from build123d import *

# Parameters (mm, degrees)
F0_W     = 254
F0_H     = 254
F1_DEPTH = 38.1
F2_SIZE  = 12.7
F3_R     = 21.5591889527
F4_DEPTH = 38.1
F5_W     = 101.6
F5_H     = 50.8
F6_DEPTH = 3.175
F7_W     = 88.9000004845
F7_H     = 38.1000004845
F8_DEPTH = 38.101
F9_R     = 5.08
F10_SIZE = 12.7


with BuildPart() as f1:
    # F0 (on Top) → F1 (new body)
    with BuildSketch(Plane.XY):
        Rectangle(F0_W, F0_H)
    extrude(amount=F1_DEPTH)

    # F2
    f2_edges = [f1.edges().sort_by_distance(p)[0] for p in [
        (-127, -127, 19.05),
        (127, -127, 19.05),
        (-127, 127, 19.05),
        (127, 127, 19.05),
    ]]
    chamfer(f2_edges, length=F2_SIZE)

    # F3 (on face) → F4 (cut, through all)
    with BuildSketch(Plane.XY.offset(38.1)):
        with Locations((0, 50.8)):
            Circle(F3_R)
    extrude(amount=-F4_DEPTH, mode=Mode.SUBTRACT)

    # F5 (on face) → F6 (cut)
    with BuildSketch(Plane.XY.offset(38.1)):
        with Locations((0, -68.0069606819)):
            Rectangle(F5_W, F5_H)
    extrude(amount=-F6_DEPTH, mode=Mode.SUBTRACT)

    # F7 (on face) → F8 (cut, through all)
    with BuildSketch(Plane.XY.offset(38.1)):
        with Locations((0, -68.0069606819)):
            Rectangle(F7_W, F7_H)
    extrude(amount=-F8_DEPTH, mode=Mode.SUBTRACT)

    # F9
    f9_edges = [f1.edges().sort_by_distance(p)[0] for p in [
        (-50.8, -42.606961, 36.5125),
        (-44.45, -48.95696, 17.4625),
        (44.45, -48.95696, 17.4625),
        (50.8, -42.606961, 36.5125),
        (50.8, -93.406961, 36.5125),
        (44.45, -87.056961, 17.4625),
        (-44.45, -87.056961, 17.4625),
        (-50.8, -93.406961, 36.5125),
    ]]
    fillet(f9_edges, radius=F9_R)

    # F10
    f10_edges = [f1.edges().sort_by_distance(p)[0] for p in [
        (0, -127, 38.1),
        (-120.65, -120.65, 38.1),
        (-127, 0, 38.1),
        (-120.65, 120.65, 38.1),
        (0, 127, 38.1),
        (120.65, 120.65, 38.1),
        (120.65, -120.65, 38.1),
        (127, 0, 38.1),
    ]]
    chamfer(f10_edges, length=F10_SIZE)


solid = f1.part
Here's how the part is built. I have some questions about the finished solid (model axes, mm). A direction names the side the tool comes from. Round coordinates to 2 decimals unless told otherwise and drop trailing zeros. Write each loop counter-clockwise with the first axis right and the second up, starting at its lowest first coordinate (ties: lowest second). Pieces come first, ordered by that corner, then holes.
1. Suppose I cut it at B-B (x = 0). List the corners of the cut face in (y, z) for me (3 decimals), and give its area (3 significant figures).
2. Suppose I cut it at D-D (x = -82.5). List the corners of the cut face in (y, z) for me, and give its area (3 significant figures).
3. I need wall thicknesses on L1, parallel to Y at x = 0, z = 9; L2, parallel to X at y = 50, z = 21; L3, parallel to Y at x = 27, z = 6. Which ranges of each line are inside material? Lowest first, please.
4. For faces 4 (the flat face through (-44.45, -68, 18)), 5 (the flat face through (0, -47, 34.925)), 6 (the flat face through (120.7, -120.6, 12.5)), which set-ups out of +Z, -Z, +X, -X, +Y, -Y let a thin tool reach every point of the face, with its end or its side?
5. Will these pins go through, and if not, where does the flat tip stop? pin 1 Ø1.6 at (y, z) = (-77, 36.5) entering from -X; pin 2 Ø2.5 at (x, z) = (-5.5, 37) entering from -Y; pin 3 Ø3.5 at (x, z) = (-20, 36.5) entering from +Y.
6. If we mould it in two halves opening along X, with no side actions, what happens to faces 1 (the flat face through (-2, 2, 0)), 2 (the flat face through (-127, -2, 13)), 3 (the flat face through (44.45, -68, 18))? For each: released by +X, released by -X, zero draft, split by the parting line, or undercut.
7. Suppose I cut it at C-C (z = 22). List the corners of the cut face in (x, y) for me.
8. Suppose I cut it at A-A (y = 50.8). List the corners of the cut face in (x, z) for me.
Answer sheet:
1. outline: (-127, 0) - (-87.057, 0) - (-87.057, 34.925) - (-93.407, 34.925) - (-93.407, 38.1) - (-114.3, 38.1) - (-127, 25.4) - close; (-48.957, 0) - (29.241, 0) - (29.241, 38.1) - (-42.607, 38.1) - (-42.607, 34.925) - (-48.957, 34.925) - close; (72.359, 0) - (127, 0) - (127, 25.4) - (114.3, 38.1) - (72.359, 38.1) - close
1. area: 6,380 mm2
2. outline: (-127, 0) - (127, 0) - (127, 25.4) - (114.3, 38.1) - (-114.3, 38.1) - (-127, 25.4) - close
2. area: 9,520 mm2
3. L1: y = -127 to -87.06, -48.96 to 29.24, 72.36 to 127
3. L2: x = -127 to -21.54, 21.54 to 127
3. L3: y = -127 to -87.06, -48.96 to 127
4. face 4: +Z, -Z
4. face 5: +Z
4. face 6: +Z, -Z, +X, -Y
5. pin 1: stops at x = -116.7
5. pin 2: stops at y = -116.65
5. pin 3: stops at y = 117.65
6. face 1: zero draft
6. face 2: released by -X
6. face 3: undercut
7. outline: (-127, -114.3) - (-114.3, -127) - (114.3, -127) - (127, -114.3) - (127, 114.3) - (114.3, 127) - (-114.3, 127) - (-127, 114.3) - close; hole (-44.45, -81.98) arc R5.08 ccw to (-39.37, -87.06) - (39.37, -87.06) arc R5.08 ccw to (44.45, -81.98) - (44.45, -54.04) arc R5.08 ccw to (39.37, -48.96) - (-39.37, -48.96) arc R5.08 ccw to (-44.45, -54.04) - close; hole circle Ø43.12 at (0, 50.8)
8. outline: (-127, 0) - (-21.56, 0) - (-21.56, 38.1) - (-114.3, 38.1) - (-127, 25.4) - close; (21.56, 0) - (127, 0) - (127, 25.4) - (114.3, 38.1) - (21.56, 38.1) - close
